```python
from build123d import *

# Parameters (mm, degrees)
SKETCH1_R               = 3.25
BOSS_EXTRUDE1_DEPTH     = 50
CHAMFER4_SIZE           = 7
CHAMFER4_SIZE2          = 10
SKETCH2_R               = 5.5
CUT_EXTRUDE1_DEPTH      = 45
CUT_EXTRUDE3_DEPTH      = 56.397262251
CUT_EXTRUDE3_DEPTH_BACK = 50
CUT_EXTRUDE4_DEPTH      = 45
CHAMFER5_SIZE           = 5
SKETCH3_R               = 0.9
CUT_EXTRUDE5_DEPTH      = 10
FILLET1_R               = 3


with BuildPart() as part:
    # Sketch1 → Boss-Extrude1 (new body)
    with BuildSketch(Plane(origin=(0, 0, 0), x_dir=(1, 0, 0), z_dir=(0, 1, 0))):
        Polygon((-5.320759509, 8), (-22.469015665, -7.56), (22.469015665, -7.56), (5.320759509, 8), align=None)
        with Locations(Location((0, 0, 0), (0, 0, 270))):
            Circle(SKETCH1_R, mode=Mode.SUBTRACT)
    extrude(amount=BOSS_EXTRUDE1_DEPTH)

    # Chamfer4
    chamfer4_edges = [part.edges().sort_by_distance(p)[0] for p in [
        (22.469015665, 25, 7.56),
    ]]
    chamfer4_side = [part.faces().sort_by_distance(p)[0] for p in [
        (0, 25, 7.56),
    ]]
    chamfer(chamfer4_edges, length=CHAMFER4_SIZE, length2=CHAMFER4_SIZE2, reference=chamfer4_side[0])

    # Sketch2 → Cut-Extrude1 (cut)
    with BuildSketch(Plane(origin=(0, 50, 0), x_dir=(1, 0, 0), z_dir=(0, 1, 0))):
        with Locations(Location((0, 0, 0), (0, 0, 270))):
            Circle(SKETCH2_R)
    extrude(amount=-CUT_EXTRUDE1_DEPTH, mode=Mode.SUBTRACT)

    # Sketch4 → Cut-Extrude3 (cut, two sides: drawn at the far end of the back side and taken through both)
    with BuildSketch(Plane.XZ.offset(-CUT_EXTRUDE3_DEPTH_BACK)):
        with BuildLine():
            Line((-6.5, 0), (-6.5, 8.455296228))
            Line((-6.5, 8.455296228), (-18.092934759, 18.509530088))
            Line((-18.092934759, 18.509530088), (-27.843988074, 13.266508324))
            Line((-27.843988074, 13.266508324), (-26.239796982, -3.957148404))
            Line((-26.239796982, -3.957148404), (-22.051551969, -11.746511534))
            Line((-22.051551969, -11.746511534), (6.44529607, -11.904202977))
            Line((6.44529607, -11.904202977), (12.131507072, -6.5))
            Line((12.131507072, -6.5), (0, -6.5))
            ThreePointArc((0, -6.5), (-4.596194078, -4.596194078), (-6.5, 0))
        make_face()
    extrude(amount=CUT_EXTRUDE3_DEPTH + CUT_EXTRUDE3_DEPTH_BACK, mode=Mode.SUBTRACT)

    # Sketch5 → Cut-Extrude4 (cut)
    with BuildSketch(Plane(origin=(0, 50, 0), x_dir=(1, 0, 0), z_dir=(0, 1, 0))):
        Polygon((0, 0), (4.867894822, -2.56), (20.482845708, -2.56), (8.2569175, 8.380042473), (1.341376292, 8.380042473), (-9.589048862, 8.380042473), (-9.589048862, -2.56), (-4.867894822, -2.56), align=None)
    extrude(amount=-CUT_EXTRUDE4_DEPTH, mode=Mode.SUBTRACT)

    # Chamfer5
    chamfer5_edges = [part.edges().sort_by_distance(p)[0] for p in [
        (10.017520214, 5, 2.56),
        (-5.683947411, 5, 2.56),
    ]]
    chamfer(chamfer5_edges, length=CHAMFER5_SIZE)

    # Sketch3 → Cut-Extrude5 (cut)
    with BuildSketch(Plane.XY.offset(7.56)):
        with Locations((12.5, 47.5)):
            Circle(SKETCH3_R)
        with Locations((12.5, 10.5)):
            Circle(SKETCH3_R)
    extrude(amount=-CUT_EXTRUDE5_DEPTH, mode=Mode.SUBTRACT)

    # Fillet1
    fillet1_edges = [part.edges().sort_by_distance(p)[0] for p in [
        (15.318080635, 50, 5.06),
        (-6.5, 50, 5.06),
    ]]
    fillet(fillet1_edges, radius=FILLET1_R)


solid = part.part
```
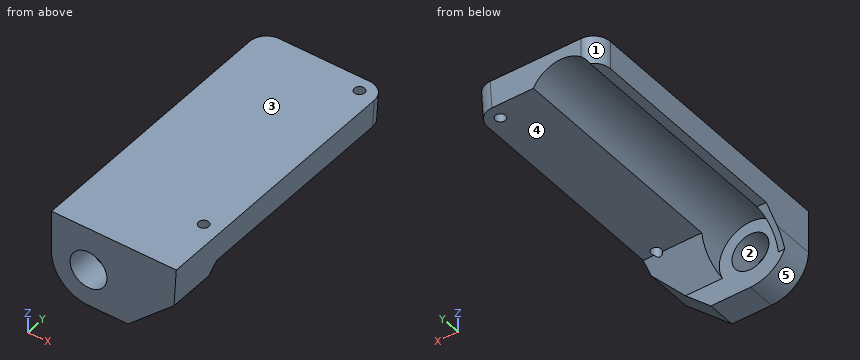
Model file for the job. Use its own axes, mm. Face numbers are marked on the shaded views. A direction names the side the tool comes from. Give positions to 0.01 mm unless a question says otherwise; leave off trailing zeros. Order: outer loops, then holes, each group sorted by start corner. A loop starts at its lowest first (then second) coordinate and runs counter-clockwise, first axis right, second up.
1) Saw through at D-D, the plane y = 45. Write the cut outline in (x, z), then the cut area to 3 significant figures.
2) 3-axis set-ups, long thin cutter, end or side, ignore diameter. For the marked faces 4 and 5: which of +Z, -Z, +X, -X, +Y, -Y reach the whole face in a straight line?
3) Saw through at A-A, the plane y = 10.5. Write the cut outline in (x, z), then the cut area to 3 significant figures.
4) Wall check: probe 1 along Y at (x, z) = (12.5, 6.2); probe 2 along X at (y, z) = (10.5, 4); probe 3 along Y at (x, z) = (-3.5, 2.5). Give the ranges that are in metal, low to high.
5) Saw through at B-B, the plane x = 1.5. Write the cut outline in (y, z).
6) Saw through at C-C, the plane z = -1. Write the cut outline in (x, y), then the cut area to 3 significant figures.
7) Mould opens along Z. For the marked faces 1, 2 and 3 say: +Z half, -Z half, draft (parallel to the pull), parting line (faces both ways), or undercut.
8) Pin check, flat tips, straight feed: pin 1 (8 mm diameter, centred on x = 11, y = 26.5, fed in from -Z); pin 2 (6 mm diameter, centred on y = 10, z = -3, fed in from +X); pin 3 (4 mm diameter, centred on y = 22, z = 2.5, fed in from +X); pin 4 (6 mm diameter, centred on y = 6, z = -5, fed in from -X). Stop position of each tip, or through.
Computed:
1. outline: (-6.5, 2.56) - (-4.87, 2.56) arc R5.5 cw to (4.87, 2.56) - (15.17, 2.56) - (15.47, 7.56) - (-6.5, 7.56) - close
1. area: 88.7 mm2
2. face 4: -Z, +X, -X, +Y
2. face 5: -Z, -X, +Y, -Y
3. outline: (-6.5, 2.56) - (-4.87, 2.56) arc R5.5 cw to (4.87, 2.56) - (11.6, 2.56) - (11.6, 7.56) - (-6.5, 7.56) - close; (13.4, 2.56) - (15.17, 2.56) - (15.47, 7.56) - (13.4, 7.56) - close
3. area: 79.7 mm2
4. probe 1: y = 0 to 9.6, 11.4 to 46.6, 48.4 to 50
4. probe 2: x = -6.5 to -3.77, 3.77 to 11.6, 13.4 to 15.25
4. probe 3: y = 0 to 5
5. outline: (0, -6.5) - (5, -6.5) - (5, -2.88) - (0, -2.88) - close; (0, 2.88) - (5, 2.88) - (5, 5.29) - (50, 5.29) - (50, 7.56) - (0, 7.56) - close
6. outline: (-6.42, 0) - (-3.09, 0) - (-3.09, 5) - (-5.41, 5) - (-5.41, 6.44) - (-6.42, 6.44) - close; (3.09, 0) - (13.04, 0) - (13.04, 6.44) - (5.41, 6.44) - (5.41, 5) - (3.09, 5) - close
6. area: 78.8 mm2
7. face 1: draft
7. face 2: undercut
7. face 3: +Z half
8. pin 1: stops at z = 2.56
8. pin 2: passes through
8. pin 3: stops at x = 15.28
8. pin 4: stops at x = -6.16
